CAD build for the part. Positions are in the model's coordinates, mm. A direction names the side the tool comes from. Coordinates: 2 decimals unless noted, no trailing zeros. Order: outer loops, then holes, each group sorted by start corner. A loop starts at its lowest first (then second) coordinate and runs counter-clockwise, first axis right, second up. Notation, with made-up numbers: (11.25, 33.5) - (38.25, 33.5) arc R30 ccw to (38.25, 64.5) - close; hole circle Ø7 at (40, 53.25). An arc over 180 degrees is marked (long way). Use one line per item in the form item = value.
```python
from build123d import *

# Parameters (mm, degrees)
F0_W     = 14.89632
F0_H     = 6.825086
F0_W_2   = 11.260638
F0_H_2   = 6.909038
F1_DEPTH = 2.54


with BuildPart() as f1:
    # F0 (on Front) → F1 (new body)
    with BuildSketch(Plane.XZ):
        Polygon((-12.7, 0), (0, 0), (12.7, 0), (12.7, 20.552527), (7.44816, 20.552527), (-7.44816, 20.552527), (-12.7, 20.552527), align=None)
        with Locations((0, 23.96507)):
            Rectangle(F0_W, F0_H)
        Polygon((-7.44816, 34.213562), (-7.44816, 27.377613), (7.44816, 27.377613), (7.44816, 34.213562), (5.630319, 34.213562), (-5.630319, 34.213562), align=None)
        with Locations((0, 37.668081)):
            Rectangle(F0_W_2, F0_H_2)
    extrude(amount=-F1_DEPTH)


solid = f1.part
```
Item 1: Cut at A-A, the plane y = 0.6. Write the cut outline in (x, z).
Derived:
outline = (-12.7, 0) - (12.7, 0) - (12.7, 20.55) - (7.45, 20.55) - (7.45, 34.21) - (5.63, 34.21) - (5.63, 41.12) - (-5.63, 41.12) - (-5.63, 34.21) - (-7.45, 34.21) - (-7.45, 20.55) - (-12.7, 20.55) - close
Item 2: Drill centre lines: line 1 (X direction, y = 0.9, z = 24); line 2 (Z direction, x = 10.5, y = 1.95); line 3 (X direction, y = 0.7, z = 39). Where is each one in solid material? Low to high. Write a range as [from, to].
Derived:
line_1 = [-7.45, 7.45]
line_2 = [0, 20.55]
line_3 = [-5.63, 5.63]
Item 3: Drop flat-ended pins along their axis: pin 1 (1.5 mm diameter, centred on x = -7, y = 1.5, fed in from +Z); pin 2 (1.3 mm diameter, centred on x = -11, y = 0.5, fed in from +Z); pin 3 (1.3 mm diameter, centred on y = 1.5, z = 38.5, fed in from -X). Give the stop position or say it passes through.
Derived:
pin_1 = 34.21
pin_2 = 20.55
pin_3 = -5.63
Item 4: 3-axis set-ups, long thin cutter, end or side, ignore diameter. For faces 1 (the face through (0, 1, 0)), 2 (the face through (-10, 1, 20.553)), 3 (the face through (7.448, 1, 27)): which of +Z, -Z, +X, -X, +Y, -Y reach the whole face in a straight line?
Derived:
face_1 = -Z, +X, -X, +Y, -Y
face_2 = +Z, -X, +Y, -Y
face_3 = +Z, +X, +Y, -Y
Item 5: Cut at C-C, the plane x = -10.75. Write the cut outline in (y, z).
Derived:
outline = (0, 0) - (2.54, 0) - (2.54, 20.55) - (0, 20.55) - close
Item 6: Cut at B-B, the plane z = 22. Write the cut outline in (x, y), plus the area to 3 significant figures.
Derived:
outline = (-7.45, 0) - (7.45, 0) - (7.45, 2.54) - (-7.45, 2.54) - close
area = 37.8 mm²
